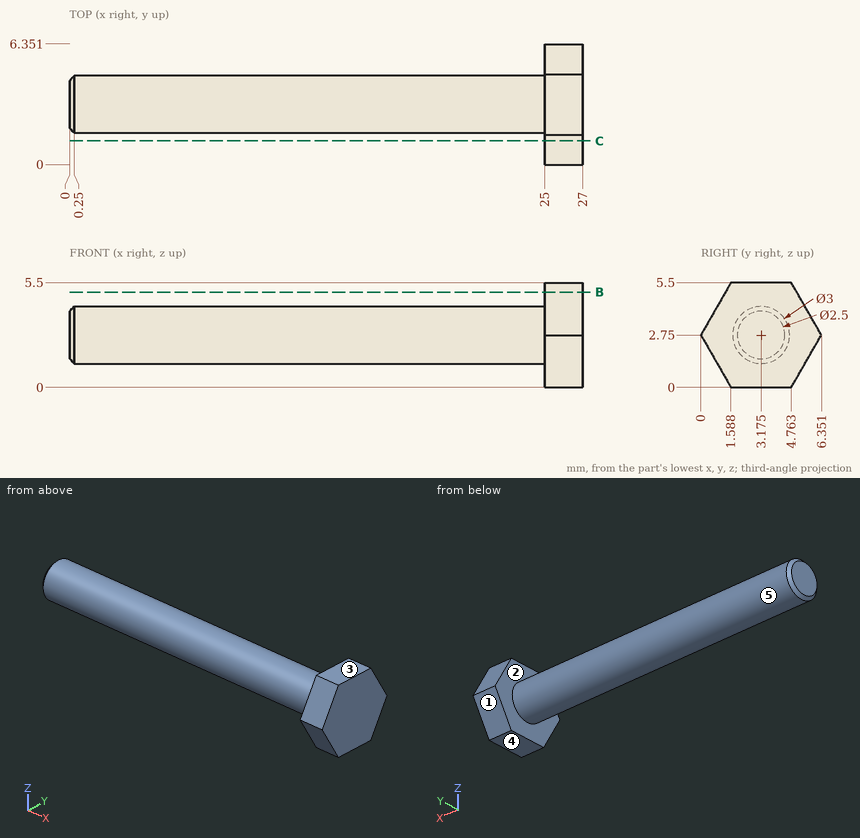
Can you work these out from the drawing? Everything is in mm from the part's minimum corner. A direction names the side the tool comes from. Coordinates: 2 decimals unless noted, no trailing zeros. Loops run counter-clockwise (first coordinate to the right, second up) from the corner with the lowest first, then second, coordinate; pieces in that order, holes last.
1) Imagine slicing it at B-B on z = 5. List the corners of the cut face in (x, y) for me.
2) I need wall thicknesses on probe 1 along X at (y, z) = (1, 1.55); probe 2 along Z at (x, y) = (18.5, 4) (1 decimal); probe 3 along Y at (x, z) = (12, 1.75) (1 decimal). Which ranges of each line are inside material? Lowest first, please.
3) Thinking about a two-plate mould opening in Z: for the marked faces 3, 4 and 5, which applies, pulls with the +Z half, pulls with the -Z half, needs draft (parallel to the pull), parting line crosses it, or undercut?
4) For pin 1 (3 mm diameter, centred on y = 2, z = 3, fed in from -X); pin 2 (2 mm diameter, centred on x = 23.5, z = 3.5, fed in from +Y) (1 decimal), each with a flat end and sliding along its axis, tell me the tip position at first contact or that it passes through.
5) Which directions (+Z, -Z, +X, -X, +Y, -Y) give clear straight access to the entire face, cutting with the end or side of a thin tool? Please do the marked faces 1 and 2.
6) Imagine slicing it at C-C on y = 1.25. List the corners of the cut face in (x, z) for me (1 decimal).
Completed:
1. outline: (25, 1.3) - (27, 1.3) - (27, 5.05) - (25, 5.05) - close
2. probe 1: x = 25 to 27
2. probe 2: z = 1.5 to 4
2. probe 3: y = 2.1 to 4.3
3. face 3: pulls with the +Z half
3. face 4: pulls with the -Z half
3. face 5: parting line crosses it
4. pin 1: stops at x = 0
4. pin 2: stops at y = 4.7
5. face 1: -Z, +X, -X, +Y
5. face 2: -X
6. outline: (25, 0.6) - (27, 0.6) - (27, 4.9) - (25, 4.9) - close
